Geometry check sheet. Reference: drawing and pictorial views, mm from the part's lowest x, y, z. A direction names the side the tool comes from. Round coordinates to 2 decimals unless told otherwise and drop trailing zeros. Order: outer loops, then holes, each group sorted by start corner. A loop starts at its lowest first (then second) coordinate and runs counter-clockwise, first axis right, second up.
(1) Cross-section at B-B on z = 5. Enter the section's corners in (x, y), and give its area (3 significant figures).
(2) Cross-section at D-D on y = 114.5. Enter the section's corners in (x, z), and give its area (3 significant figures).
(3) Draft check along Y on the marked faces 3, 4, 5 and 6. Enter one of: pulls with the +Y half, pulls with the -Y half, needs draft (parallel to the pull), parting line crosses it, or undercut.
(4) Thickness scan on L1, parallel to Y at x = 55, z = 22.75; L2, parallel to Y at x = 32.5, z = 2; L3, parallel to Y at x = 190, z = 20.5. Record the ranges inside material, lowest first.
(5) Cross-section at A-A on x = 55. Enter the section's corners in (y, z), and give its area (3 significant figures).
(6) Gauge pin test, flat ends, axial feed: P1, Ø1.5, axis at x = 130.5, y = 51, coming from the -Z side; P2, Ø3.5, axis at x = 52.5, y = 23.5, coming from the +Z side; P3, Ø7.5, axis at y = 118, z = 13.5, coming from the -X side. Record the tip position at first contact, or that the pin passes through.
(7) Set-up check for the marked faces 1 and 2: record each of +Z, -Z, +X, -X, +Y, -Y from which the full face is reachable in a straight line by a thin tool's end or side.
(8) Cross-section at C-C on y = 226. Enter the section's corners in (x, z), and give its area (3 significant figures).
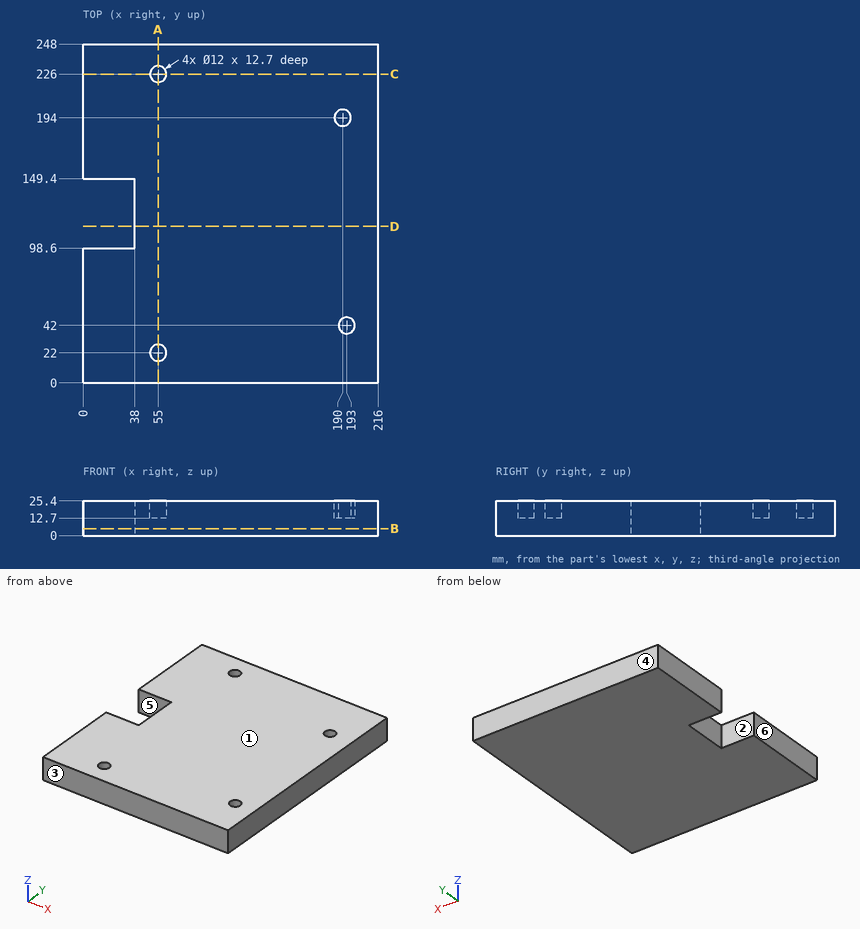
Found:
1. outline: (0, 0) - (216, 0) - (216, 248) - (0, 248) - (0, 149.4) - (38, 149.4) - (38, 98.6) - (0, 98.6) - close
1. area: 51,600 mm2
2. outline: (38, 0) - (216, 0) - (216, 25.4) - (38, 25.4) - close
2. area: 4,520 mm2
3. face 3: pulls with the -Y half
3. face 4: pulls with the +Y half
3. face 5: undercut
3. face 6: needs draft
4. L1: y = 0 to 16, 28 to 220, 232 to 248
4. L2: y = 0 to 98.6, 149.4 to 248
4. L3: y = 0 to 36.8, 47.2 to 188, 200 to 248
5. outline: (0, 0) - (248, 0) - (248, 25.4) - (232, 25.4) - (232, 12.7) - (220, 12.7) - (220, 25.4) - (28, 25.4) - (28, 12.7) - (16, 12.7) - (16, 25.4) - (0, 25.4) - close
5. area: 5,990 mm2
6. P1: stops at z = 0
6. P2: stops at z = 12.7
6. P3: stops at x = 38
7. face 1: +Z, +X, -X, +Y, -Y
7. face 2: +Z, -Z, -X
8. outline: (0, 0) - (216, 0) - (216, 25.4) - (61, 25.4) - (61, 12.7) - (49, 12.7) - (49, 25.4) - (0, 25.4) - close
8. area: 5,330 mm2
